Build history of the part. All positions in model axes, mm. A direction names the side the tool comes from. Round coordinates to 2 decimals unless told otherwise and drop trailing zeros. Order: outer loops, then holes, each group sorted by start corner. A loop starts at its lowest first (then second) coordinate and runs counter-clockwise, first axis right, second up. Notation, with made-up numbers: M 20.25,72 L 77.25,72 A21 cw 77.25,98 Z; hole C 8.5,0 d8. An arc over 180 degrees is marked long. One line per item, written item: value. Start each with the question number.
Item 1: Band-saw the part on A-A, the plane y = -18. Write the cut outline in (x, z), then the cut area to 3 significant figures.
Item 2: Band-saw the part on B-B, the plane x = -62. Write the cut outline in (y, z).
Item 3: Pin check, flat tips, straight feed: pin 1 (1.5 mm diameter, centred on y = -18, z = -13, fed in from -X); pin 2 (1 mm diameter, centred on x = -72.5, z = -12.5, fed in from -Y). Stop position of each tip, or through.
Item 4: Tool access for faces 4 (the flat face through (-41, -5, 35)), 5 (the flat face through (-8, -19, 0)): list every direction of +Z, -Z, +X, -X, +Y, -Y with a clear straight run to the whole face (end or side of a thin tool).
Item 5: Band-saw the part on C-C, the plane z = 15. Write the cut outline in (x, y).
Item 6: Two-plate mould, pull along X, no slides. Class faces 1 (the cylindrical face through (-80.95, -4.06, 19.22)), 2 (the flat face through (-90, -4, 0)), 3 (the flat face through (-4, -30, 0)): +X half, -X half, draft (parallel to the pull), parting line (faces both ways), or undercut.
Item 7: Probe L1, parallel to Z at x = -75, y = -1.25; L2, parallel to Z at x = -3.5, y = -18; L3, parallel to Y at x = -3, z = 15. List the from-to ranges inside material, lowest first.
Item 8: Band-saw the part on D-D, the plane z = 6.5. Write the cut outline in (x, y), then the cut area to 3 significant figures.
Autodesk Inventor part; units mm, degrees
ref_plane "YZ Plane" through (0, 0, 0) normal (1, 0, 0) x (0, 1, 0)
ref_plane "XZ Plane" through (0, 0, 0) normal (0, 1, 0) x (-1, 0, 0)
ref_plane "XY Plane" through (0, 0, 0) normal (0, 0, 1) x (1, 0, 0)
sketch "Esboço1" plane through (0, 0, 0) normal (0, 0, 1) x (1, 0, 0)
  line L0 (-90, 0) -> (0, 0)
  line L1 (0, 0) -> (0, -30)
  line L2 (0, -30) -> (-8, -30)
  line L3 (-8, -30) -> (-8, -8)
  line L4 (-8, -8) -> (-90, -8)
  line L5 (-90, -8) -> (-90, 0)
  dimension "d0" = 90
  dimension "d1" = 30
  dimension "d2" = 8
  dimension "d3" = 8
extrude "Extrusão1" add sketch "Esboço1" along normal mid plane 70
sketch "Esboço2" plane through (-90, 0, 35) normal (0, 1, 0) x (1, 0, 0)
  line L0 (0, 70) -> (0, 0)
  line L1 (90, 0) -> (0, 0)
  line L2 (0, 70) -> (90, 70)
  point P0 (90, 35)
  point P1 (28, 55)
  point P2 (15, 15)
  dimension "d6" = 28
  dimension "d7" = 15
  dimension "d8" = 15
  dimension "d9" = 15
hole "Furo1" at (-62, 0, -20) at (-75, 0, 20) direction (0, -1, 0) diameter 12 end through all
sketch "Esboço3" plane through (-8, -30, 35) normal (-1, 0, 0) x (0, 0, 1)
  line L0 (-70, 0) -> (0, 0)
  line L1 (0, 22) -> (0, 0)
  line L2 (-70, 0) -> (-70, 22)
  point P0 (-35, 30)
  point P1 (-50, 12)
  point P2 (-20, 12)
  dimension "d17" = 12
  dimension "d18" = 20
  dimension "d19" = 20
hole "Furo2" at (-8, -18, -15) at (-8, -18, 15) direction (1, 0, 0) diameter 4.5 end through all
chamfer "Chanfro1" distance 10 angle 45 4 edges at (-90, -4, -35) (-90, -4, 35) (-4, -30, -35) (-4, -30, 35)
Output:
1. outline: M -8,-35 L 0,-35 L 0,-17.25 L -8,-17.25 Z; M -8,-12.75 L 0,-12.75 L 0,12.75 L -8,12.75 Z; M -8,17.25 L 0,17.25 L 0,35 L -8,35 Z
1. area: 488 mm²
2. outline: M -8,-35 L 0,-35 L 0,-26 L -8,-26 Z; M -8,-14 L 0,-14 L 0,35 L -8,35 Z
3. pin 1: stops at x = -8
3. pin 2: stops at y = -8
4. face 4: +Z, +X, -X, +Y, -Y
4. face 5: +Z, -Z, -X, -Y
5. outline: M -90,-8 L -78.32,-8 L -78.32,0 L -90,0 Z; M -71.68,-8 L -8,-8 L -8,-15.75 L 0,-15.75 L 0,0 L -71.68,0 Z; M -8,-30 L 0,-30 L 0,-20.25 L -8,-20.25 Z
6. face 1: undercut
6. face 2: -X half
6. face 3: draft
7. L1: z = -35 to 14, 26 to 35
7. L2: z = -35 to -17.25, -12.75 to 12.75, 17.25 to 35
7. L3: y = -30 to -20.25, -15.75 to 0
8. outline: M -90,-8 L -8,-8 L -8,-30 L 0,-30 L 0,0 L -90,0 Z
8. area: 896 mm²
